```python
from build123d import *

# Parameters (mm, degrees)
F0_W     = 76.2
F0_H     = 76.2
F1_DEPTH = 76.2
F2_R     = 26.969245
F3_DEPTH = 76.201
F4_SIZE  = 5.08


with BuildPart() as f1:
    # F0 (on Front) → F1 (new body)
    with BuildSketch(Plane.XZ):
        with Locations((0.212106, -0.679574)):
            Rectangle(F0_W, F0_H)
    extrude(amount=F1_DEPTH)

    # F2 (on face) → F3 (cut, through all)
    with BuildSketch(Plane(origin=(0, 0, 0), x_dir=(-1, 0, 0), z_dir=(0, 1, 0))):
        with Locations((-1.895509, -2.46492)):
            Circle(F2_R)
    extrude(amount=-F3_DEPTH, mode=Mode.SUBTRACT)

    # F4
    f4_edges = [f1.edges().sort_by_distance(p)[0] for p in [
        (-37.887894, -38.1, 37.420426),
        (-37.887894, -38.1, -38.779574),
        (-37.887894, 0, -0.679574),
        (-37.887894, -76.2, -0.679574),
        (38.312106, -38.1, -38.779574),
        (0.212106, 0, -38.779574),
        (0.212106, -76.2, -38.779574),
        (38.312106, -38.1, 37.420426),
        (38.312106, 0, -0.679574),
        (38.312106, -76.2, -0.679574),
        (0.212106, 0, 37.420426),
        (0.212106, -76.2, 37.420426),
    ]]
    chamfer(f4_edges, length=F4_SIZE)


solid = f1.part
```
Part model, mm, in its own coordinate system. Give positions to 0.01 mm unless a question says otherwise; leave off trailing zeros. Order: outer loops, then holes, each group sorted by start corner. A loop starts at its lowest first (then second) coordinate and runs counter-clockwise, first axis right, second up. Notation, with made-up numbers: (13.25, 45.25) - (43.25, 45.25) arc R20 cw to (43.25, 79.25) - close; hole circle Ø10 at (29, -36). An arc over 180 degrees is marked (long way). Use one line per item in the form item = value.
Item 1: Probe probe 1 along X at (y, z) = (-20, -2); probe 2 along Z at (x, y) = (-9.5, -24.5); probe 3 along X at (y, z) = (-44, 22). List the from-to ranges inside material, lowest first. Write a range as from..to.
Solution:
probe_1 = -37.89..-25.07, 28.86..38.31
probe_2 = -38.78..-26.91, 21.98..37.42
probe_3 = -37.89..-9.45, 13.24..38.31
Item 2: Slice it at B-B on z = 18.5. Give the cut face in (x, y).
Solution:
outline = (-37.89, -71.12) - (-32.81, -76.2) - (-15.07, -76.2) - (-15.07, 0) - (-32.81, 0) - (-37.89, -5.08) - close; (18.86, -76.2) - (33.23, -76.2) - (38.31, -71.12) - (38.31, -5.08) - (33.23, 0) - (18.86, 0) - close
Item 3: Slice it at C-C on y = -34. Give the cut face in (x, z), and give its area (3 significant figures).
Solution:
outline = (-37.89, -33.7) - (-32.81, -38.78) - (33.23, -38.78) - (38.31, -33.7) - (38.31, 32.34) - (33.23, 37.42) - (-32.81, 37.42) - (-37.89, 32.34) - close; hole circle Ø53.94 at (1.9, -2.46)
area = 3,470 mm2
Item 4: Two-plate mould, pull along Z, no slides. Class faces 1 (the face through (-37.888, -38, -1)), 2 (the face through (-23.02, -37.57, -12.79)), 3 (the face through (-34.413, -3.14, 33.875)): released by +Z, released by -Z, zero draft, split by the parting line, or undercut.
Solution:
face_1 = zero draft
face_2 = undercut
face_3 = released by +Z
Item 5: Slice it at A-A on x = 22.5. Give the cut face in (y, z), and give its area (3 significant figures).
Solution:
outline = (-76.2, -33.7) - (-71.12, -38.78) - (-5.08, -38.78) - (0, -33.7) - (0, -19.87) - (-76.2, -19.87) - close; (-76.2, 14.94) - (0, 14.94) - (0, 32.34) - (-5.08, 37.42) - (-71.12, 37.42) - (-76.2, 32.34) - close
area = 3,100 mm2
